Source: CAD feature listing. Evaluate the final solid. Frame: model axes, mm. Round coordinates to 2 decimals unless told otherwise and drop trailing zeros. Write each loop counter-clockwise with the first axis right and the second up, starting at its lowest first coordinate (ties: lowest second). Pieces come first, ordered by that corner, then holes. Notation, with made-up numbers: M -22,84 L 1,84 A20 cw 1,103 Z; hole C -36.5,-6.75 d4. An arc over 180 degrees is marked long. Use a Markdown table: item, result.
```python
from build123d import *

# Parameters (mm, degrees)
F0_R     = 1.4
F0_W     = 6.426
F0_H     = 20.883
F1_DEPTH = 0.5


with BuildPart() as f1:
    # F0 (on Front) → F1 (new body)
    with BuildSketch(Plane.XZ):
        Polygon((-32.8, -45.3), (32.8, -45.3), (32.8, 17.52029), (32.8, 38.40329), (32.8, 45.3), (-32.8, 45.3), align=None)
        with Locations((-31.1, -34.3)):
            Circle(F0_R, mode=Mode.SUBTRACT)
        with Locations((29.4, -43.4)):
            Circle(F0_R, mode=Mode.SUBTRACT)
        with Locations((-30.4, 42.9)):
            Circle(F0_R, mode=Mode.SUBTRACT)
        with Locations((29.4, 42.1)):
            Circle(F0_R, mode=Mode.SUBTRACT)
        with Locations((36.013, 27.96179)):
            Rectangle(F0_W, F0_H)
    extrude(amount=F1_DEPTH)


solid = f1.part
```
Q1. Line query: L1, parallel to Z at x = 29.4, y = -0.1; L2, parallel to X at y = -0.1, z = -28. Output: solid intervals per line, ascending.
Results are:
| item | result |
|---|---|
| L1 | -45.3 to -44.8, -42 to 40.7, 43.5 to 45.3 |
| L2 | -32.8 to 32.8 |
Q2. Section C-C on y = -0.4. Return loops of the section in (x, z), plus the area to 3 significant figures.
Results are:
| item | result |
|---|---|
| outline | M -32.8,-45.3 L 32.8,-45.3 L 32.8,17.52 L 39.23,17.52 L 39.23,38.4 L 32.8,38.4 L 32.8,45.3 L -32.8,45.3 Z; hole C -31.1,-34.3 d2.8; hole C -30.4,42.9 d2.8; hole C 29.4,-43.4 d2.8; hole C 29.4,42.1 d2.8 |
| area | 6,050 mm^2 |
Q3. First-contact query: pin 1 Ø4.5 at (x, z) = (-30.4, 42.9) entering from +Y; pin 2 Ø1.7 at (x, z) = (29.4, -43.4) entering from +Y. Flat tips, straight axial feed; report the tip coordinate or a pass-through.
Results are:
| item | result |
|---|---|
| pin 1 | y = 0 |
| pin 2 | through |
Q4. Section A-A on x = 29.4. Return loops of the section in (y, z), plus the area to 3 significant figures.
Results are:
| item | result |
|---|---|
| outline | M -0.5,-45.3 L 0,-45.3 L 0,-44.8 L -0.5,-44.8 Z; M -0.5,-42 L 0,-42 L 0,40.7 L -0.5,40.7 Z; M -0.5,43.5 L 0,43.5 L 0,45.3 L -0.5,45.3 Z |
| area | 42.5 mm^2 |
Q5. Section B-B on z = -43.4. Return loops of the section in (x, y).
Results are:
| item | result |
|---|---|
| outline | M -32.8,-0.5 L 28,-0.5 L 28,0 L -32.8,0 Z; M 30.8,-0.5 L 32.8,-0.5 L 32.8,0 L 30.8,0 Z |
Q6. Section D-D on z = -18.5. Return loops of the section in (x, y).
Results are:
| item | result |
|---|---|
| outline | M -32.8,-0.5 L 32.8,-0.5 L 32.8,0 L -32.8,0 Z |
Q7. Mould query, pull axis X, two halves, no side actions, for faces 1 (the flat face through (3, -0.5, 1)), 2 (the cylindrical face through (-30.35, -0.25, -33.12)). Classes: +X half, -X half, draft (parallel to the pull), parting line (faces both ways), or undercut.
Results are:
| item | result |
|---|---|
| face 1 | draft |
| face 2 | undercut |
